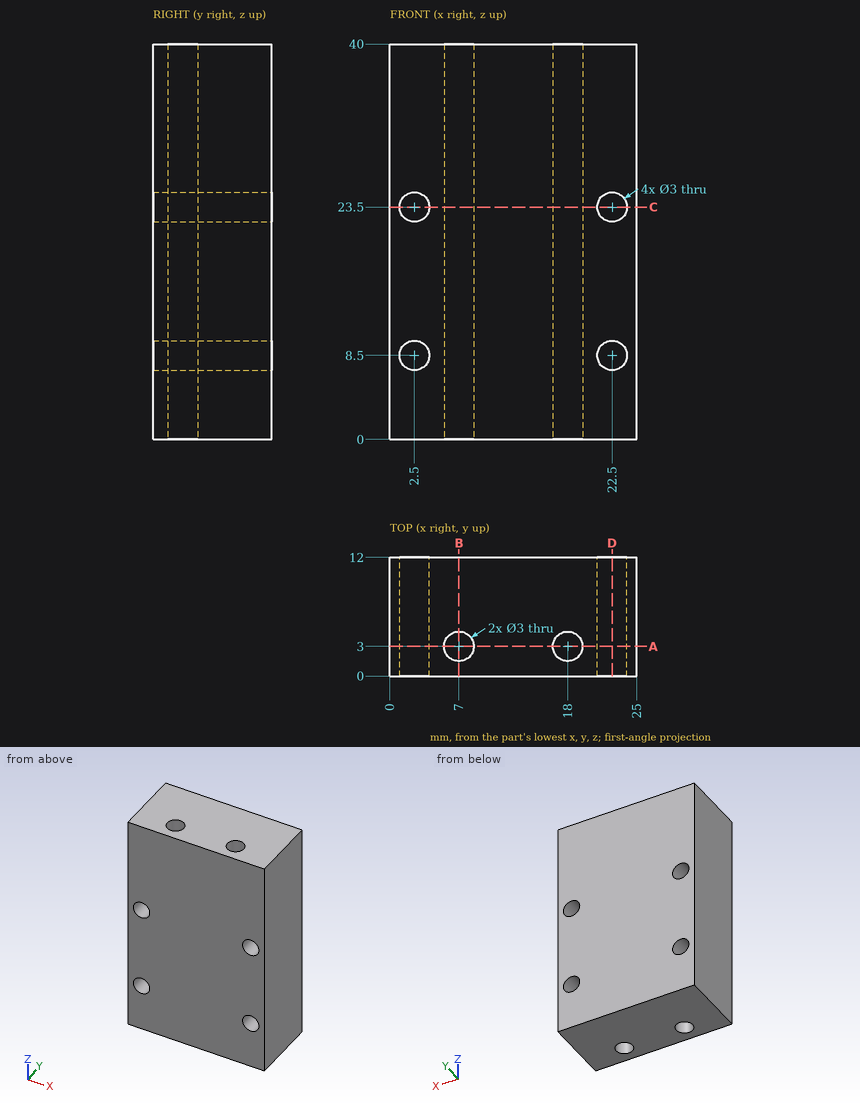
Geometry check sheet. Reference: drawing and pictorial views, mm from the part's lowest x, y, z. Round coordinates to 2 decimals unless told otherwise and drop trailing zeros. Order: outer loops, then holes, each group sorted by start corner. A loop starts at its lowest first (then second) coordinate and runs counter-clockwise, first axis right, second up. Notation, with made-up numbers: (14, 40) - (26, 40) arc R17 ccw to (26, 73) - close; hole circle Ø3 at (71, 42.5). An arc over 180 degrees is marked (long way). Use a Markdown table: item, result. Add a question column.
1) Section check C-C (z = 23.5). Record the cut outline in (x, y).
2) Section check B-B (x = 7). Record the cut outline in (y, z).
3) Thickness scan on line 1 along Z through (x, y) = (2.5, 4); line 2 along X through (y, z) = (8, 23); line 3 along Y through (x, z) = (18, 17). Record the ranges inside material, lowest first.
4) Section check D-D (x = 22.5). Record the cut outline in (y, z), then the cut area to 3 significant figures.
5) Section check A-A (y = 3). Record the cut outline in (x, z).
6) Gauge pin test, flat end, axial feed: P1, Ø1.8, axis at x = 18, y = 3, coming from the +Z side. Record the tip position at first contact, or that the pin passes through.
Established:
| question | item | result |
|---|---|---|
| 1 | outline | (0, 0) - (1, 0) - (1, 12) - (0, 12) - close; (4, 0) - (21, 0) - (21, 12) - (4, 12) - close; (24, 0) - (25, 0) - (25, 12) - (24, 12) - close; hole circle Ø3 at (7, 3); hole circle Ø3 at (18, 3) |
| 2 | outline | (0, 0) - (1.5, 0) - (1.5, 40) - (0, 40) - close; (4.5, 0) - (12, 0) - (12, 40) - (4.5, 40) - close |
| 3 | line 1 | 0 to 7, 10 to 22, 25 to 40 |
| 3 | line 2 | 0 to 1.09, 3.91 to 21.09, 23.91 to 25 |
| 3 | line 3 | 0 to 1.5, 4.5 to 12 |
| 4 | outline | (0, 0) - (12, 0) - (12, 7) - (0, 7) - close; (0, 10) - (12, 10) - (12, 22) - (0, 22) - close; (0, 25) - (12, 25) - (12, 40) - (0, 40) - close |
| 4 | area | 408 mm2 |
| 5 | outline | (0, 0) - (5.5, 0) - (5.5, 40) - (0, 40) - close; (8.5, 0) - (16.5, 0) - (16.5, 40) - (8.5, 40) - close; (19.5, 0) - (25, 0) - (25, 40) - (19.5, 40) - close; hole circle Ø3 at (2.5, 8.5); hole circle Ø3 at (2.5, 23.5); hole circle Ø3 at (22.5, 8.5); hole circle Ø3 at (22.5, 23.5) |
| 6 | P1 | through |
